Autodesk Inventor part; units mm, degrees
ref_plane "YZ Plane" through (0, 0, 0) normal (1, 0, 0) x (0, 1, 0)
ref_plane "XZ Plane" through (0, 0, 0) normal (0, 1, 0) x (-1, 0, 0)
ref_plane "XY Plane" through (0, 0, 0) normal (0, 0, 1) x (1, 0, 0)
sketch "スケッチ1" plane through (0, 0, 0) normal (0, 0, 1) x (1, 0, 0)
  circle A0 centre (0, 0) radius 10
  circle A1 centre (0, 0) radius 9
  line L0 (-14, 0) -> (14, 0) construction
  line L1 (0, -14) -> (0, 14) construction
  circle A2 centre (-6, 0) radius 2.05
  circle A3 centre (6, 0) radius 2.05
  dimension "d0" = 20
  dimension "d1" = 18
  dimension "d2" = 4.1
  dimension "d3" = 6
extrude "押し出し1" add sketch "スケッチ1" along normal blind 9 contours A0 | A1 | A2 | A3
extrude "押し出し2" cut sketch "スケッチ1" along normal blind 2 contours A1
extrude "押し出し4" add sketch "スケッチ1" against normal blind 0.88 contours A2 | A3
chamfer "面取り1" distance 0.3 angle 45 2 edges at (-8.05, 0, -0.88) (3.95, 0, -0.88)
properties part number "wheel"
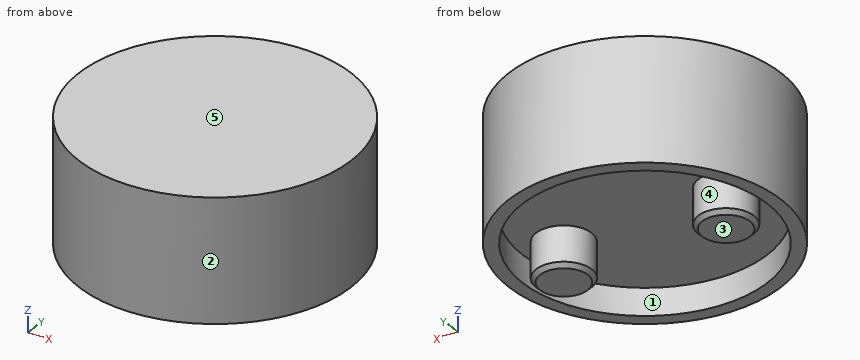
Read the model definition and answer for the solid it produces. Units are mm, in the model's axes. Face numbers are marked on the shaded views. A direction names the side the tool comes from. Round coordinates to 2 decimals unless told otherwise and drop trailing zeros. Order: outer loops, then holes, each group sorted by start corner. A loop starts at its lowest first (then second) coordinate and runs counter-clockwise, first axis right, second up.
1) For the marked faces 4 and 5, determine the directions among +Z, -Z, +X, -X, +Y, -Y from which every point of the face is accessible in a straight line to the end or side of a thin tool.
2) A flat-ended cylindrical pin translates along its axis: pin 1 (10 mm diameter, centred on x = -0.5, y = 5, fed in from -Z). Find the tip coordinate at first contact, or state that the pin passes through.
3) Straight lines are drawn through the part: L1, parallel to Y at x = 0, z = 0.8; L2, parallel to X at y = 1.5, z = 0.5; L3, parallel to Z at x = 2.5, y = 8.5. For each, find the intervals that lie inside material, in ascending order.
4) The mould has two halves that part along Y. Classify the marked faces 1, 2 and 3: released by +Y, released by -Y, zero draft, split by the parting line, or undercut.
5) The part is cut by section C-C on y = 0. Write down the section's boundary in (x, z), plus the area to 3 significant figures.
6) The part is cut by section D-D on z = 6.5. Write down the section's boundary in (x, y).
7) The part is cut by section B-B on z = 1. Write down the section's boundary in (x, y), plus the area to 3 significant figures.
8) The part is cut by section A-A on x = 0. Write down the section's boundary in (y, z).
Resolved:
1. face 4: -Z
1. face 5: +Z, +X, -X, +Y, -Y
2. pin 1: stops at z = 0
3. L1: y = -10 to -9, 9 to 10
3. L2: x = -9.89 to -8.87, -7.4 to -4.6, 4.6 to 7.4, 8.87 to 9.89
3. L3: z = 2 to 9
4. face 1: undercut
4. face 2: split by the parting line
4. face 3: zero draft
5. outline: (-10, 0) - (-9, 0) - (-9, 2) - (-8.05, 2) - (-8.05, -0.58) - (-7.75, -0.88) - (-4.25, -0.88) - (-3.95, -0.58) - (-3.95, 2) - (3.95, 2) - (3.95, -0.58) - (4.25, -0.88) - (7.75, -0.88) - (8.05, -0.58) - (8.05, 2) - (9, 2) - (9, 0) - (10, 0) - (10, 9) - (-10, 9) - close
5. area: 167 mm2
6. outline: circle Ø20 at (0, 0)
7. outline: circle Ø20 at (0, 0); circle Ø4.1 at (-6, 0); circle Ø4.1 at (6, 0); hole circle Ø18 at (0, 0)
7. area: 86.1 mm2
8. outline: (-10, 0) - (-9, 0) - (-9, 2) - (9, 2) - (9, 0) - (10, 0) - (10, 9) - (-10, 9) - close
